For this review, take the finished solid that the model builds, in its own axes (mm). Face numbers are marked on the shaded views. Round coordinates to 2 decimals unless told otherwise and drop trailing zeros. Order: outer loops, then holes, each group sorted by start corner. A loop starts at its lowest first (then second) coordinate and runs counter-clockwise, first axis right, second up. Notation, with made-up numbers: M 13.25,33.5 L 37.25,33.5 A19 ccw 37.25,45.5 Z; hole C -40,64.5 d6. An arc over 180 degrees is marked long. Answer as a JSON object with one key per item and string values.
from build123d import *

# Parameters (mm, degrees)
SKIZZE1_R                       = 1.7
AUFSATZ_LINEAR_AUSTRAGEN1_DEPTH = 6
SKIZZE2_R                       = 4
SCHNITT_LINEAR_AUSTRAGEN1_DEPTH = 0.5
SKIZZE3_R                       = 3
SCHNITT_LINEAR_AUSTRAGEN2_DEPTH = 2


with BuildPart() as part:
    # Skizze1 → Aufsatz-Linear austragen1 (new body)
    with BuildSketch(Plane.XY):
        with BuildLine():
            Line((-49.2275, -51.8905), (-49.2275, -56.581162408))
            ThreePointArc((-49.2275, -56.581162408), (-50.407885162, -59.393344486), (-53.227421196, -60.556054132))
            Line((-53.227421196, -60.556054132), (-175.420431309, -60.556054132))
            ThreePointArc((-175.420431309, -60.556054132), (-177.965722471, -59.641745773), (-179.34742314, -57.316800583))
            Line((-179.34742314, -57.316800583), (-179.34742314, -52.3842))
            ThreePointArc((-179.34742314, -52.3842), (-176.514207067, -44.783915623), (-169.0581, -41.5905))
            Line((-169.0581, -41.5905), (-59.5275, -41.5905))
            ThreePointArc((-59.5275, -41.5905), (-52.244300154, -44.607300154), (-49.2275, -51.8905))
        make_face()
        with Locations((-55.2338, -48.0905)):
            Circle(SKIZZE1_R, mode=Mode.SUBTRACT)
        with Locations((-172.84742314, -48.0905)):
            Circle(SKIZZE1_R, mode=Mode.SUBTRACT)
    extrude(amount=AUFSATZ_LINEAR_AUSTRAGEN1_DEPTH)

    # Skizze2 → Schnitt-Linear austragen1 (cut)
    with BuildSketch(Plane.XY.offset(6)):
        with Locations((-152.34742314, -51.0905)):
            Circle(SKIZZE2_R)
        with Locations(Location((-76.269564564, -51.215358923, 0), (0, 0, 180))):
            Circle(SKIZZE2_R)
    extrude(amount=-SCHNITT_LINEAR_AUSTRAGEN1_DEPTH, mode=Mode.SUBTRACT)

    # Skizze3 → Schnitt-Linear austragen2 (cut)
    with BuildSketch(Plane.XY.offset(6)):
        with Locations((-172.84742314, -48.0905)):
            Circle(SKIZZE3_R)
        with Locations((-55.2338, -48.0905)):
            Circle(SKIZZE3_R)
    extrude(amount=-SCHNITT_LINEAR_AUSTRAGEN2_DEPTH, mode=Mode.SUBTRACT)


solid = part.part
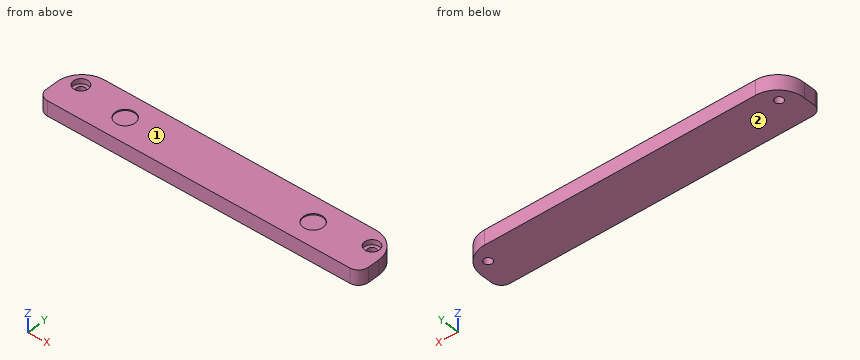
1) For L1, parallel to X at y = -48, z = 4.7; L2, parallel to X at y = -52.5, z = 0.55; L3, parallel to X at y = -48.5, z = 4.2, list the stretches that pass through material, from the lowest coordinate up.
Geometry check:
{"L1": "x = -178.6 to -175.85, -169.85 to -58.23, -52.24 to -49.99", "L2": "x = -179.35 to -49.23", "L3": "x = -178.78 to -175.82, -169.88 to -58.21, -52.26 to -49.8"}
2) Insertion check: P1, Ø2.5, axis at x = -152.5, y = -49.5, coming from the +Z side; P2, Ø1, axis at y = -46.5, z = 4, coming from the -X side; P3, Ø3, axis at x = -54.5, y = -47.5, coming from the +Z side. Each pin has a flat end and moves straight along its axis. Give the tip position at first contact, or say it passes through.
Geometry check:
{"P1": "stops at z = 5.5", "P2": "stops at x = -178.12", "P3": "stops at z = 4"}
3) Mouldability with a two-part tool opening along Z and no side actions: class the marked faces 1 and 2 as +Z half, -Z half, draft (parallel to the pull), parting line (faces both ways), or undercut.
Geometry check:
{"face 1": "+Z half", "face 2": "-Z half"}
4) Add section B-B on x = -149.5. State the section outline as (y, z) points.
Geometry check:
{"outline": "M -60.56,0 L -41.59,0 L -41.59,6 L -48.28,6 L -48.28,5.5 L -53.9,5.5 L -53.9,6 L -60.56,6 Z"}
5) Add section A-A on z = 1.65. State the section outline as (x, y) points, and give its area (3 significant figures).
Geometry check:
{"outline": "M -179.35,-57.32 A4 ccw -175.42,-60.56 L -53.23,-60.56 A4 ccw -49.23,-56.58 L -49.23,-51.89 A10.3 ccw -59.53,-41.59 L -169.06,-41.59 A10.3 ccw -179.35,-52.38 Z; hole C -172.85,-48.09 d3.4; hole C -55.23,-48.09 d3.4", "area": "2,400 mm²"}
